from build123d import *

# Parameters (mm, degrees)
EXTRUDE_THIN1_DEPTH = 400


with BuildPart() as part:
    # Sketch1 → Extrude-Thin1 (new body)
    with BuildSketch(Plane(origin=(0, 0, 0), x_dir=(1, 0, 0), z_dir=(0, 1, 0))):
        with BuildLine():
            Line((-46.726101212, 151.113189738), (-6.724981576, 151.113189738))
            ThreePointArc((-6.724981576, 151.113189738), (-3.011728055, 149.461688161), (-1.751349164, 145.598120611))
            Line((-1.751349164, 145.598120611), (-2.499982506, -54.513654379))
            ThreePointArc((-2.499982506, -54.513654379), (1.362139111, -62.445932955), (10.001711114, -64.233339564))
            Line((10.001711114, -64.233339564), (49.661853535, -64.233339564))
            Line((49.661853535, -64.233339564), (49.661853535, -59.233339564))
            Line((49.661853535, -59.233339564), (9.254697404, -59.233339564))
            ThreePointArc((9.254697404, -59.233339564), (4.6438767, -58.655180628), (2.499982506, -54.532359627))
            Line((2.499982506, -54.532359627), (3.247845267, 145.373437083))
            ThreePointArc((3.247845267, 145.373437083), (0.603039342, 152.9177067), (-6.724981576, 156.113189738))
            Line((-6.724981576, 156.113189738), (-46.726101212, 156.113189738))
            Line((-46.726101212, 156.113189738), (-46.726101212, 151.113189738))
        make_face()
    extrude(amount=EXTRUDE_THIN1_DEPTH)


solid = part.part
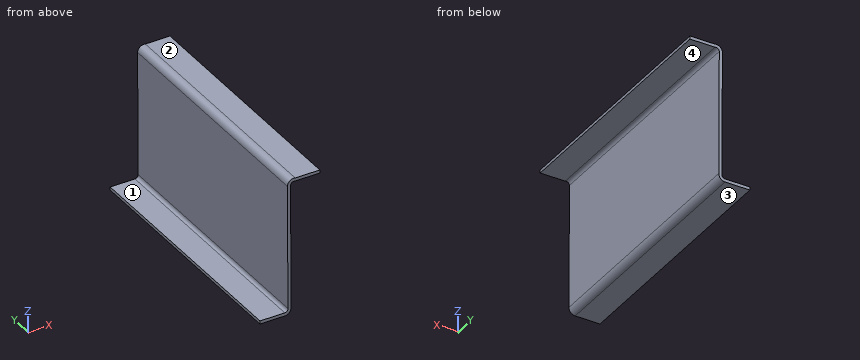
Geometry: final body of the model. Coordinates: model frame, mm. Face numbers are marked on the shaded views. A direction names the side the tool comes from. Give positions to 0.01 mm unless a question says otherwise; leave off trailing zeros. Order: outer loops, then holes, each group sorted by start corner. A loop starts at its lowest first (then second) coordinate and runs counter-clockwise, first axis right, second up. Notation, with made-up numbers: (55, 87.25) -> (103, 87.25) arc R13 ccw to (103, 102.25) -> close; hole circle Ø2 at (36, -3). An arc over 180 degrees is marked (long way). Write each question's results on one line, items separated by ' | '.
1) Cut plane C-C (z = -36). Output: boundary loops of the cut face in (x, y).
Geometry says:
outline: (-2.16, 0) -> (2.84, 0) -> (2.84, 400) -> (-2.16, 400) -> close
2) First-contact query: pin 1 Ø4 at (y, z) = (131, -64) entering from -X; pin 2 Ø10 at (x, y) = (39.5, 347.5) entering from -Z; pin 3 Ø8 at (x, z) = (8.5, 28.5) entering from -Y; pin 4 Ø12 at (x, y) = (-1, 58.5) entering from +Z. Flat tips, straight axial feed; report the tip coordinate or a pass-through.
Geometry says:
pin 1: stops at x = -2.06 | pin 2: stops at z = 59.23 | pin 3: passes through | pin 4: stops at z = 64.23
3) Cut plane B-B (x = 14). Output: boundary loops of the cut face in (y, z).
Geometry says:
outline: (0, 59.23) -> (400, 59.23) -> (400, 64.23) -> (0, 64.23) -> close
4) Cut plane A-A (y = 284). Output: boundary loops of the cut face in (x, z).
Geometry says:
outline: (-46.73, -156.11) -> (-6.72, -156.11) arc R10 ccw to (3.25, -145.37) -> (2.5, 54.53) arc R5 cw to (9.25, 59.23) -> (49.66, 59.23) -> (49.66, 64.23) -> (10, 64.23) arc R10 ccw to (-2.5, 54.51) -> (-1.75, -145.6) arc R5 cw to (-6.72, -151.11) -> (-46.73, -151.11) -> close
5) Line query: line 1 along Z through (x, y) = (-11, 51); line 2 along X through (y, z) = (260, -128); line 3 along Z through (x, y) = (32.5, 87). Output: solid intervals per line, ascending.
Geometry says:
line 1: z = -156.11 to -151.11 | line 2: x = -1.82 to 3.18 | line 3: z = 59.23 to 64.23
6) Set-up query: the marked faces 1, 2, 3 and 4. Return all of +Z, -Z, +X, -X, +Y, -Y with unobstructed straight access to the full face (end or side cutting, diameter ignored); none if empty.
Geometry says:
face 1: +Z, -X, +Y, -Y | face 2: +Z, +X, +Y, -Y | face 3: -Z, +X, -X, +Y, -Y | face 4: -Z, +X, +Y, -Y
